For this review, take the finished solid that the model builds, in its own axes (mm). A direction names the side the tool comes from. Give positions to 0.01 mm unless a question says otherwise; leave off trailing zeros. Write each loop counter-clockwise with the first axis right and the second up, starting at its lowest first coordinate (ties: lowest second). Pieces come first, ordered by that corner, then holes. Notation, with made-up numbers: M 8,26 L 19,26 A34 ccw 19,59 Z; hole C 60.25,36.5 d11. An arc over 180 degrees is marked long. One line per item, written item: value. Start each with the question number.
Item 1: Consider section A-A, the plane z = 59. Write out the cut boundary in (x, y), and give its area (3 significant figures).
Item 2: Mouldability with a two-part tool opening along Z and no side actions: class faces 1 (the face through (5.045, 0.493, -115.302)), 2 (the face through (8, 1, 3)) as released by +Z, released by -Z, zero draft, split by the parting line, or undercut.
Item 3: Tool access review of faces 3 (the face through (-5.045, 0.493, 115.302)), 4 (the face through (8, 0, 3)): name each direction out of +Z, -Z, +X, -X, +Y, -Y from which nothing blocks a thin tool from reaching the whole face with its end or side.
Item 4: To check wall thickness, follow probe 1 along X at (y, z) = (0.5, -157.5); probe 2 along X at (y, z) = (0.85, -30); probe 3 along X at (y, z) = (0.7, 178.5). State the ranges of each line that lie inside material, in increasing order.
Item 5: Consider section B-B, the plane y = 0.5. Give the number of separate pieces and of enclosed holes in the cut face, and give its area (3 significant figures).
Item 6: Clearance check with flat-ended pins moving along their axes: pin 1 Ø3 at (x, z) = (27, -116.5) entering from -Y; pin 2 Ø3.5 at (x, z) = (-32.4, -127.5) entering from +Y; pin 3 Ø0.5 at (y, z) = (0.5, -164.5) entering from -X. State where each tip first meets the part, or that it passes through.
```python
from build123d import *

# Parameters (mm, degrees)
SKETCH1_R           = 2.15
SKETCH1_W           = 13.8
SKETCH1_H           = 239
BOSS_EXTRUDE1_DEPTH = 1
FILLET2_R           = 10


with BuildPart() as part:
    # Sketch1 → Boss-Extrude1 (new body)
    with BuildSketch(Plane(origin=(0, 0, 0), x_dir=(1, 0, 0), z_dir=(0, 1, 0))):
        Polygon((-39.9, -163.5), (-21.9, -163.5), (-21.9, -167.5), (-16.9, -167.5), (-16.9, -183.5), (16.9, -183.5), (16.9, -167.5), (21.9, -167.5), (21.9, -163.5), (39.9, -163.5), (39.9, 163.5), (21.9, 163.5), (21.9, 167.5), (16.9, 167.5), (16.9, 183.5), (-16.9, 183.5), (-16.9, 167.5), (-21.9, 167.5), (-21.9, 163.5), (-39.9, 163.5), align=None)
        with Locations(Location((-32.4, 127.5, 0), (0, 0, 270))):
            Circle(SKETCH1_R, mode=Mode.SUBTRACT)
        with Locations(Location((32.4, 127.5, 0), (0, 0, 270))):
            Circle(SKETCH1_R, mode=Mode.SUBTRACT)
        with Locations(Location((-32.4, -127.5, 0), (0, 0, 270))):
            Circle(SKETCH1_R, mode=Mode.SUBTRACT)
        with Locations(Location((32.4, -127.5, 0), (0, 0, 270))):
            Circle(SKETCH1_R, mode=Mode.SUBTRACT)
        with Locations(Location((-32.4, -157.5, 0), (0, 0, 270))):
            Circle(SKETCH1_R, mode=Mode.SUBTRACT)
        with Locations(Location((32.4, -157.5, 0), (0, 0, 270))):
            Circle(SKETCH1_R, mode=Mode.SUBTRACT)
        with Locations(Location((32.4, 157.5, 0), (0, 0, 270))):
            Circle(SKETCH1_R, mode=Mode.SUBTRACT)
        with Locations(Location((-32.4, 157.5, 0), (0, 0, 270))):
            Circle(SKETCH1_R, mode=Mode.SUBTRACT)
        with Locations(Location((0, 178.5, 0), (0, 0, 270))):
            Circle(SKETCH1_R, mode=Mode.SUBTRACT)
        with Locations(Location((0, -178.5, 0), (0, 0, 270))):
            Circle(SKETCH1_R, mode=Mode.SUBTRACT)
        Rectangle(SKETCH1_W, SKETCH1_H, mode=Mode.SUBTRACT)
    extrude(amount=BOSS_EXTRUDE1_DEPTH)

    # Fillet2
    # the kernel refuses this fillet: 10 mm, written as the material it adds along each edge
    with BuildSketch(Plane(origin=(6.9, 0, -119.5), x_dir=(-1, 0, 0), z_dir=(0, 1, 0)), Plane(origin=(6.9, 0, 119.5), x_dir=(0, 0, -1), z_dir=(0, 1, 0)), Plane(origin=(-6.9, 0, 119.5), x_dir=(1, 0, 0), z_dir=(0, 1, 0))) as fillet2_piece_1:
        with BuildLine():
            CenterArc((FILLET2_R, FILLET2_R), FILLET2_R, 180, 90)
            Line((0, FILLET2_R), (0, 0))
            Line((0, 0), (FILLET2_R, 0))
        make_face()
    extrude(amount=1)
    with BuildSketch(Plane(origin=(-6.9, 0, -119.5), x_dir=(1, 0, 0), z_dir=(0, 1, 0))) as fillet2_piece_2:
        with BuildLine():
            CenterArc((FILLET2_R, -FILLET2_R), FILLET2_R, 90, 90)
            Line((0, -FILLET2_R), (0, 0))
            Line((0, 0), (FILLET2_R, 0))
        make_face()
    extrude(amount=1)


solid = part.part
```
Model answer:
1. outline: M -39.9,0 L -6.9,0 L -6.9,1 L -39.9,1 Z; M 6.9,0 L 39.9,0 L 39.9,1 L 6.9,1 Z
1. area: 66.0 mm2
2. face 1: undercut
2. face 2: zero draft
3. face 3: +Y, -Y
3. face 4: +Z, -Z, +X, -X, -Y
4. probe 1: x = -39.9 to -34.55, -30.25 to 30.25, 34.55 to 39.9
4. probe 2: x = -39.9 to -6.9, 6.9 to 39.9
4. probe 3: x = -16.9 to -2.15, 2.15 to 16.9
5. separate pieces: 1
5. enclosed holes: 11
5. area: 24,200 mm2
6. pin 1: stops at y = 0
6. pin 2: passes through
6. pin 3: stops at x = -21.9
